```python
from build123d import *

# Parameters (mm, degrees)
SKETCH1_R               = 1.984375
BOSS_EXTRUDE1_DEPTH     = 169.87265999999997
CUT_EXTRUDE1_DEPTH      = 23.05812
CUT_EXTRUDE2_START      = -169.87266
CUT_EXTRUDE2_DEPTH      = 23.05812
FILLET1_R               = 7.62
CUT_EXTRUDE3_DEPTH      = 198.3909425992125
CUT_EXTRUDE3_DEPTH_BACK = 198.3909425992125
SKETCH6_R               = 2.000000000000001
SKETCH6_R_2             = 2.0000000000000004
CUT_EXTRUDE4_DEPTH      = 198.3909425992125
CUT_EXTRUDE4_DEPTH_BACK = 198.3909425992125
SKETCH7_W               = 96.26632678346117
SKETCH7_H               = 127.9185977098139
SKETCH7_H_2             = 40.36656229018607


with BuildPart() as part:
    # Sketch1 → Boss-Extrude1 (new body)
    with BuildSketch(Plane(origin=(0, 0, 0), x_dir=(1, 0, 0), z_dir=(0, 1, 0))):
        with BuildLine():
            Line((-9.955287346489113, -3.6074515728352274), (-6.769721367669625, -3.607451572835229))
            Line((-6.769721367669625, -3.607451572835229), (8.985913588520251, -3.607451572835254))
            Line((8.985913588520251, -3.607451572835254), (12.171479567676489, -3.6074515728352536))
            add(Edge.make_bspline(
                [(10.60289964969583, -20.752451572835255), (11.099968974105764, -15.73020157118813), (11.63056361676114, -10.016003165571298), (12.113997871046978, -4.296816952278091), (12.171479567676489, -3.6074515728352536)],
                knots=[0.38496962590391054, 0.38496962590391054, 0.38496962590391054, 0.38496962590391054, 0.4581086713676085, 0.468131593311824, 0.468131593311824, 0.468131593311824, 0.468131593311824], degree=3))
            add(Edge.make_bspline(
                [(1.1080961105936413, -99.87377835629641), (4.527344743513003, -73.53176416291807), (7.98655990047842, -47.18721965154313), (10.60289964969583, -20.752451572835255)],
                knots=[0, 0, 0, 0, 0.38496962590391054, 0.38496962590391054, 0.38496962590391054, 0.38496962590391054], degree=3))
            add(Edge.make_bspline(
                [(1.1080961105936413, -99.87377835629641), (-2.311152522316452, -73.53176416292023), (-5.77036767929202, -47.18721965154205), (-8.386707428509173, -20.752451572835213)],
                knots=[0, 0, 0, 0, 0.3849696259039116, 0.3849696259039116, 0.3849696259039116, 0.3849696259039116], degree=3))
            add(Edge.make_bspline(
                [(-8.386707428509173, -20.752451572835213), (-8.88377675291906, -15.730201571188243), (-9.414371395575616, -10.016003165551764), (-9.897805649859515, -4.296816952279357), (-9.955287346489113, -3.6074515728352274)],
                knots=[0.3849696259039116, 0.3849696259039116, 0.3849696259039116, 0.3849696259039116, 0.4581086713676079, 0.46813159331185, 0.46813159331185, 0.46813159331185, 0.46813159331185], degree=3))
        make_face()
        with Locations(Location((1.10810856874065, -11.326456678177, 0), (0, 0, 270))):
            Circle(SKETCH1_R, mode=Mode.SUBTRACT)
    extrude(amount=BOSS_EXTRUDE1_DEPTH)

    # Sketch2 → Cut-Extrude1 (cut)
    with BuildSketch(Plane(origin=(0, 169.87265999999997, 0), x_dir=(1, 0, 0), z_dir=(0, 1, 0))):
        Polygon((-9.955287346489113, -3.6074515728352274), (25.808519749497883, -3.6074515728352274), (25.808519749497883, -26.312456678177), (-9.95528734648911, -26.312456678177), align=None)
    extrude(amount=-CUT_EXTRUDE1_DEPTH, mode=Mode.SUBTRACT)

    # Sketch2<2> → Cut-Extrude2 (cut)
    with BuildSketch(Plane(origin=(0, 169.87265999999997, 0), x_dir=(1, 0, 0), z_dir=(0, 1, 0)).offset(CUT_EXTRUDE2_START)):
        Polygon((-9.955287346489113, -3.6074515728352274), (25.808519749497883, -3.6074515728352274), (25.808519749497883, -26.312456678177), (-9.95528734648911, -26.312456678177), align=None)
    extrude(amount=CUT_EXTRUDE2_DEPTH, mode=Mode.SUBTRACT)

    # Fillet1
    fillet1_edges = [part.edges().sort_by_distance(p)[0] for p in [
        (-7.8241553741226255, 11.529059999999971, 26.312456678177),
        (10.040347595309392, 11.529059999999971, 26.312456678177),
        (-9.955287346489113, 84.93632999999997, 3.6074515728352274),
        (12.171479567676489, 84.93632999999997, 3.6074515728352536),
        (-7.8241553741226255, 158.34359999999998, 26.312456678177),
        (10.040347595309392, 158.34359999999998, 26.312456678177),
    ]]
    fillet(fillet1_edges, radius=FILLET1_R)

    # Sketch6 → Cut-Extrude3 (cut, two sides: drawn at the far end of the back side and taken through both)
    with BuildSketch(Plane.XZ.offset(-CUT_EXTRUDE3_DEPTH_BACK)):
        with Locations(Location((1.1080961105936413, 71.9337783562964, 0), (0, 0, 270))):
            Circle(SKETCH6_R)
        with Locations(Location((1.1080961105935272, 34.76055213743882, 0), (0, 0, 270))):
            Circle(SKETCH6_R_2)
    extrude(amount=CUT_EXTRUDE3_DEPTH + CUT_EXTRUDE3_DEPTH_BACK, mode=Mode.SUBTRACT)

    # Sketch7 → Cut-Extrude4 (cut, two sides: drawn at the far end of the back side and taken through both)
    with BuildSketch(Plane(origin=(0, 0, 0), x_dir=(0, 0, -1), z_dir=(1, 0, 0)).offset(-CUT_EXTRUDE4_DEPTH_BACK)):
        with Locations((-51.740614964565815, 63.95929885490695)):
            Rectangle(SKETCH7_W, SKETCH7_H)
        with Locations((-51.740614964565815, 149.68937885490692)):
            Rectangle(SKETCH7_W, SKETCH7_H_2)
    extrude(amount=CUT_EXTRUDE4_DEPTH + CUT_EXTRUDE4_DEPTH_BACK, mode=Mode.SUBTRACT)


solid = part.part
```
For this review, take the finished solid that the model builds, in its own axes (mm). Round coordinates to 2 decimals unless told otherwise and drop trailing zeros.
(1) Mouldability with a two-part tool opening along X and no side actions: class faces 1 (the cylindrical face through (2.46, 128.72, 73.41)), 2 (the cylindrical face through (2.46, 128.723, 36.235)), 3 (the flat face through (1, 127.919, 42)) as released by +X, released by -X, zero draft, split by the parting line, or undercut.
Returned:
face 1: undercut
face 2: undercut
face 3: zero draft
(2) We need section A-A (y = 128.7). State how many separate pieces and enclosed holes the cut face has, plus the area to 3 significant figures.
Returned:
separate pieces: 1
enclosed holes: 3
area: 1,070 mm2
(3) Wall thickness on line 1 along X through (y, z) = (128.75, 12); line 2 along X through (y, z) = (128.25, 13); line 3 along X through (y, z) = (128.7, 46): over which ranges is each line inside the solid? List them lowest first.
Returned:
line 1: x = -9.22 to -0.76, 2.97 to 11.44
line 2: x = -9.13 to 0.04, 2.17 to 11.34
line 3: x = -5.66 to 7.87
